Source: CAD feature listing. Evaluate the final solid. Frame: model axes, mm. A direction names the side the tool comes from. Give positions to 0.01 mm unless a question says otherwise; leave off trailing zeros. Order: outer loops, then holes, each group sorted by start corner. A loop starts at its lowest first (then second) coordinate and runs counter-clockwise, first axis right, second up. Notation, with made-up numbers: (-19.5, 59.5) -> (0.5, 59.5) arc R22 ccw to (0.5, 78.5) -> close; hole circle Ø3 at (19.5, 13.5). An arc over 180 degrees is marked (long way). Answer in a Markdown table with one row per item.
```python
from build123d import *

# Parameters (mm, degrees)
MODEL_R                 = 5
SALIENTE_EXTRUIR1_DEPTH = 3


with BuildPart() as part:
    # Model → Saliente-Extruir1 (new body)
    with BuildSketch(Plane.XY):
        Polygon((4.111589817, 100.015674998), (4.111565333, -10.669034302), (4.111569102, -24.246637901), (15.911569751, -24.246637901), (15.911569751, -47.446638901), (4.111568751, -47.446638901), (4.111568751, -54.531377488), (31.918927332, -54.54545045), (31.918927332, -58.038983798), (40.118927332, -58.038983798), (40.118927332, -54.538983798), (50.918927332, -54.538983798), (50.918927332, -58.038983798), (59.118927332, -58.038983798), (59.118927332, -54.538983798), (87.018940879, -54.546637), (87.018940879, -47.446639), (75.218940879, -47.446639), (75.218940879, -24.246638), (87.018940879, -24.246638), (87.111592427, 100.015659295), align=None)
        with Locations((44.026491998, -32.632550575)):
            Circle(MODEL_R, mode=Mode.SUBTRACT)
        Polygon((25.045319697, -23.106306752), (25.052514337, -17.106311065), (20.552517572, -17.100915085), (20.562110425, -9.100920836), (25.06210719, -9.106316817), (25.06930183, -3.10632113), (36.069293922, -3.119511304), (36.062099282, -9.11950699), (40.562096047, -9.12490297), (40.552503193, -17.124897219), (36.052506429, -17.119501239), (36.045311789, -23.119496925), align=None, mode=Mode.SUBTRACT)
        Polygon((66.030211381, -23.130879389), (66.030211381, -17.130879389), (70.530211381, -17.130879389), (70.530211381, -9.130879389), (66.030211381, -9.130879389), (66.030211381, -3.130879389), (55.030211381, -3.130879389), (55.030211381, -9.130879389), (50.530211381, -9.130879389), (50.530211381, -17.130879389), (55.030211381, -17.130879389), (55.030211381, -23.130879389), align=None, mode=Mode.SUBTRACT)
    extrude(amount=SALIENTE_EXTRUIR1_DEPTH)


solid = part.part
```
(1) Section query B-B (y = -6). Return the cut outline in (x, z), plus the area to 3 significant figures.
A:
| item | result |
|---|---|
| outline | (4.11, 0) -> (25.07, 0) -> (25.07, 3) -> (4.11, 3) -> close; (36.07, 0) -> (55.03, 0) -> (55.03, 3) -> (36.07, 3) -> close; (66.03, 0) -> (87.03, 0) -> (87.03, 3) -> (66.03, 3) -> close |
| area | 183 mm^2 |
(2) First-contact query: pin 1 Ø1.5 at (x, z) = (67.5, 1) entering from -Y; pin 2 Ø1.5 at (x, z) = (59.5, 1) entering from -Y; pin 3 Ø1.5 at (y, z) = (-20.5, 1.5) entering from +X; pin 4 Ø1.5 at (y, z) = (70.5, 2.5) entering from +X. Flat tips, straight axial feed; report the tip coordinate or a pass-through.
A:
| item | result |
|---|---|
| pin 1 | stops at y = -54.54 |
| pin 2 | stops at y = -58.04 |
| pin 3 | stops at x = 87.02 |
| pin 4 | stops at x = 87.09 |
(3) Ray query, probe 1 along X at (y, z) = (-16, 1.1); probe 2 along Y at (x, z) = (31, 2.3); probe 3 along Y at (x, z) = (76, 0.3). Return the intervals inside material, ascending.
A:
| item | result |
|---|---|
| probe 1 | x = 4.11 to 20.55, 40.55 to 50.53, 70.53 to 87.03 |
| probe 2 | y = -54.54 to -23.11, -3.11 to 100.02 |
| probe 3 | y = -54.54 to -47.45, -24.25 to 100.02 |
(4) Pull-direction query (X, two-part tool) for faces 1 (the flat face through (68, -9.131, 1)), 2 (the flat face through (10, -47.447, 1)), 3 (the flat face through (4.112, -51, 1)), 4 (the flat face through (53, -9.131, 1)); classes: +X half, -X half, draft (parallel to the pull), parting line (faces both ways), or undercut.
A:
| item | result |
|---|---|
| face 1 | undercut |
| face 2 | draft |
| face 3 | -X half |
| face 4 | undercut |
(5) Access query for faces 5 (the flat face through (66.03, -20, 1)), 6 (the flat face through (59.119, -56, 1)), 7 (the flat face through (81, -47.447, 1)). Directions: +Z, -Z, +X, -X, +Y, -Y. A direction counts if a zero-diameter tool reaches every point of the face in a straight line with its end or side. Return the directions, or none.
A:
| item | result |
|---|---|
| face 5 | +Z, -Z |
| face 6 | +Z, -Z, +X, -Y |
| face 7 | +Z, -Z, +X |
(6) Section query D-D (z = 0.85). Give the number of separate pieces and of enclosed holes in the cut face, plus the area to 3 significant figures.
A:
| item | result |
|---|---|
| separate pieces | 1 |
| enclosed holes | 3 |
| area | 11,700 mm^2 |
(7) Section query A-A (x = 57.5). Return the cut outline in (y, z), plus the area to 3 significant figures.
A:
| item | result |
|---|---|
| outline | (-58.04, 0) -> (-23.13, 0) -> (-23.13, 3) -> (-58.04, 3) -> close; (-3.13, 0) -> (100.02, 0) -> (100.02, 3) -> (-3.13, 3) -> close |
| area | 414 mm^2 |
(8) Section query C-C (x = 26.5). Return the cut outline in (y, z).
A:
| item | result |
|---|---|
| outline | (-54.54, 0) -> (-23.11, 0) -> (-23.11, 3) -> (-54.54, 3) -> close; (-3.11, 0) -> (100.02, 0) -> (100.02, 3) -> (-3.11, 3) -> close |
